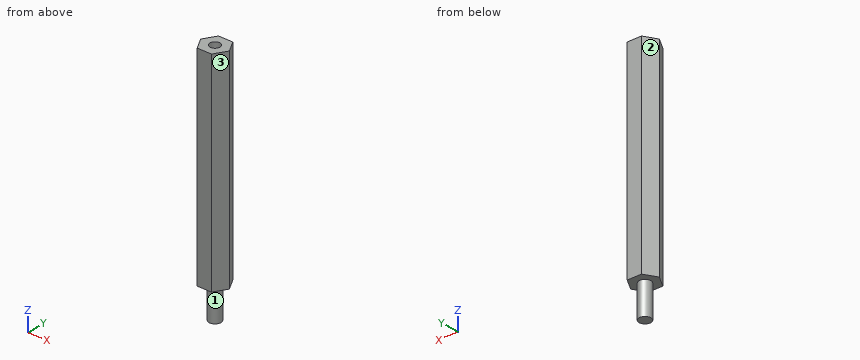
Autodesk Inventor part; units mm, degrees
ref_plane "Plan YZ" through (0, 0, 0) normal (1, 0, 0) x (0, 1, 0)
ref_plane "Plan XZ" through (0, 0, 0) normal (0, 1, 0) x (-1, 0, 0)
ref_plane "Plan XY" through (0, 0, 0) normal (0, 0, 1) x (1, 0, 0)
sketch "Esquisse1" plane through (0, 0, 0) normal (0, 0, 1) x (1, 0, 0)
  circle A0 centre (0, 0) radius 1.425
  dimension "d0" = 2.85
extrude "Extrusion1" add sketch "Esquisse1" along normal blind 7.8
sketch "Esquisse6" plane through (0, 0, 7.8) normal (0, 0, 1) x (1, 0, 0)
  line L0 (-4.8497, 0) -> (4.8497, 0) construction
  line L1 (0, -4.2) -> (0, 4.2) construction
  line L2 (-1.7321, -3) -> (-3.4641, 0)
  line L3 (-3.4641, 0) -> (-1.7321, 3)
  line L4 (-1.7321, 3) -> (0, 3)
  line L5 (-1.7321, -3) -> (0, -3)
  line L6 (1.7321, -3) -> (3.4641, 0)
  line L7 (3.4641, 0) -> (1.7321, 3)
  line L8 (1.7321, 3) -> (0, 3)
  line L9 (1.7321, -3) -> (0, -3)
  point P0 (0, 0)
  dimension "d4" = 6
  dimension "d8" = 120
  dimension "d10" = 6
extrude "Extrusion2" add sketch "Esquisse6" along normal blind 50
sketch "Esquisse7" plane through (0, 0, 57.8) normal (0, 0, 1) x (1, 0, 0)
  circle A0 centre (0, 0) radius 1.425
thread "Filetage1"
hole "Perçage1" at (0, 0, 57.8) direction (0, 0, -1) diameter 2.459 depth 8.5 tip angle 118
properties part number "entretoiseM3x50" material "."
Part model, mm, in its own coordinate system. Face numbers are marked on the shaded views. Coordinates: 2 decimals unless noted, no trailing zeros. Order: outer loops, then holes, each group sorted by start corner. A loop starts at its lowest first (then second) coordinate and runs counter-clockwise, first axis right, second up. Notation, with made-up numbers: (16, 61) - (20, 61) arc R19 ccw to (20, 77) - close; hole circle Ø2 at (4, 3). An arc over 180 degrees is marked (long way). Return JSON: item names as keys, results as strings. Group by question number.
Item 1: Pin check, flat tips, straight feed: pin 1 (3 mm diameter, centred on y = 1, z = 39, fed in from +X); pin 2 (4 mm diameter, centred on x = -2, z = 36.5, fed in from -Y); pin 3 (2 mm diameter, centred on x = 0, y = 0, fed in from +Z). Stop position of each tip, or through.
Item 2: Drill centre lines: probe 1 along X at (y, z) = (0, 52.75); probe 2 along Y at (x, z) = (0, 56); probe 3 along Y at (x, z) = (2.75, 22). Where is each one in solid material? Low to high. Write a range as from..to.
Item 3: Cut at A-A (z = 5.5). List the corners of the cut face in (x, y) (3 decimals).
Item 4: Cut at D-D (y = 2). List the corners of the cut face in (x, z).
Item 5: Cut at C-C (z = 29). List the corners of the cut face in (x, y), plus the area to 3 significant figures.
Item 6: Cut at B-B (y = -2.25). List the corners of the cut face in (x, z), plus the area to 3 significant figures.
Item 7: Pull direction Y, two halves, no side cores. Call the marked faces 1, 2 and 3: pulls with the +Y half, pulls with the -Y half, needs draft (parallel to the pull), parting line crosses it, or undercut.
Check values:
{
 "1": {"pin 1": "stops at x = 3.46", "pin 2": "stops at y = -3", "pin 3": "stops at z = 49.16"},
 "2": {"probe 1": "x = -3.46..-1.23, 1.23..3.46", "probe 2": "y = -3..-1.23, 1.23..3", "probe 3": "y = -1.24..1.24"},
 "3": {"outline": "circle Ø2.85 at (0, 0)"},
 "4": {"outline": "(-2.31, 7.8) - (2.31, 7.8) - (2.31, 57.8) - (-2.31, 57.8) - close"},
 "5": {"outline": "(-3.46, 0) - (-1.73, -3) - (1.73, -3) - (3.46, 0) - (1.73, 3) - (-1.73, 3) - close", "area": "31.2 mm2"},
 "6": {"outline": "(-2.17, 7.8) - (2.17, 7.8) - (2.17, 57.8) - (-2.17, 57.8) - close", "area": "217 mm2"},
 "7": {"face 1": "parting line crosses it", "face 2": "pulls with the +Y half", "face 3": "pulls with the -Y half"}
}
